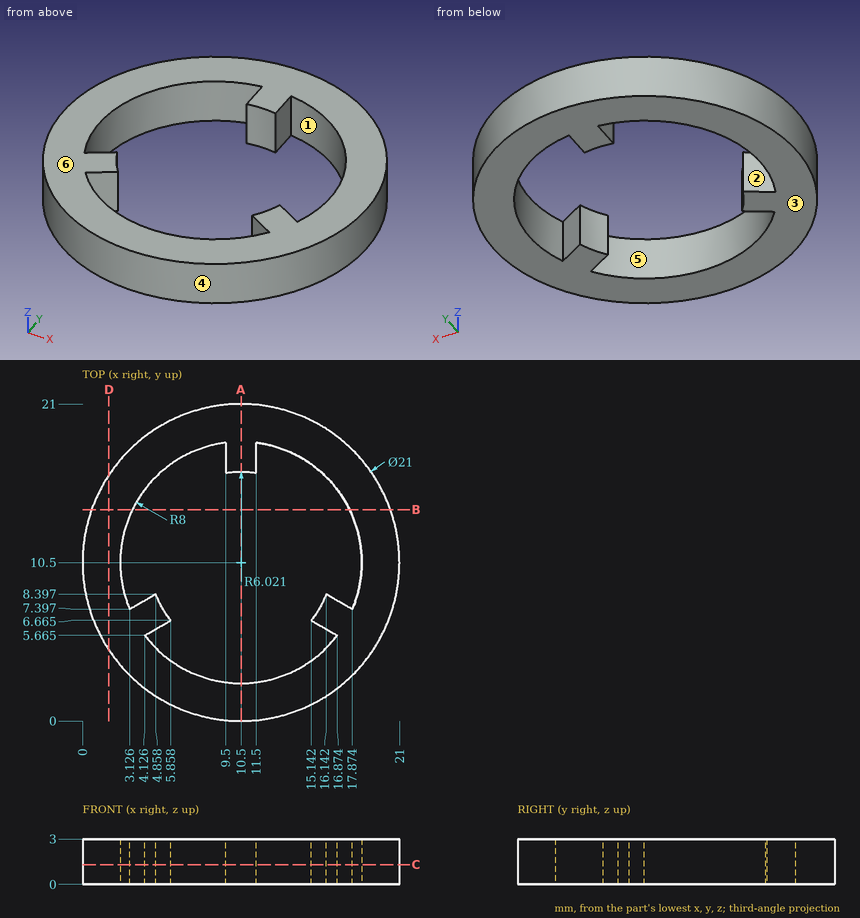
Job drawing, mm, ordinate dimensions from the low corner. One solid piece. A direction names the side the tool comes from. Round coordinates to 2 decimals unless told otherwise and drop trailing zeros. Loops run counter-clockwise (first coordinate to the right, second up) from the corner with the lowest first, then second, coordinate; pieces in that order, holes last.
(1) Cut at C-C (z = 1.3). Give the cut face in (x, y) (1 decimal).
(2) Wall check: line 1 along Y through (x, z) = (15.25, 1.85) (1 decimal); line 2 along X through (y, z) = (17.75, 0.6) (1 decimal); line 3 along Y through (x, z) = (4.75, 1.35) (1 decimal). Give the ranges that are in metal, low to high.
(3) Cut at B-B (y = 14). Give the cut face in (x, z).
(4) Cut at A-A (x = 10.5). Give the cut face in (y, z).
(5) Drop flat-ended pins along their axis: pin 1 (1.5 mm diameter, centred on x = 17, y = 14, fed in from +Z); pin 2 (1.6 mm diameter, centred on y = 18, z = 1, fed in from -X) (1 decimal); pin 3 (1 mm diameter, centred on y = 17.5, z = 1.5, fed in from +X) (1 decimal). Give the stop position or say it passes through.
(6) Two-plate mould, pull along X, no slides. Class the marked faces 1, 2, 3 and 4: +X half, -X half, draft (parallel to the pull), parting line (faces both ways), or undercut.
(7) Which spindle directions (+Z, -Z, +X, -X, +Y, -Y) get a long thin tool onto all of the face, cutting with end or side? Do the marked faces 5 and 6. Say none if no direction does.
(8) Cut at D-D (x = 1.75). Give the cut face in (y, z), plus the area to 3 significant figures.
Findings below:
1. outline: circle Ø21 at (10.5, 10.5); hole (3.1, 7.4) - (4.9, 8.4) arc R6 ccw to (5.9, 6.7) - (4.1, 5.7) arc R8 ccw to (16.9, 5.7) - (15.1, 6.7) arc R6 ccw to (16.1, 8.4) - (17.9, 7.4) arc R8 ccw to (11.5, 18.4) - (11.5, 16.4) arc R6 ccw to (9.5, 16.4) - (9.5, 18.4) arc R8 ccw to start
2. line 1: y = 1.1 to 4.1, 6.6 to 6.8, 16.9 to 19.9
2. line 2: x = 2.9 to 7.1, 9.5 to 11.5, 13.9 to 18.1
2. line 3: y = 1.7 to 4.9, 6 to 8.3, 16.1 to 19.3
3. outline: (0.6, 0) - (3.31, 0) - (3.31, 3) - (0.6, 3) - close; (17.69, 0) - (20.4, 0) - (20.4, 3) - (17.69, 3) - close
4. outline: (0, 0) - (2.5, 0) - (2.5, 3) - (0, 3) - close; (16.52, 0) - (21, 0) - (21, 3) - (16.52, 3) - close
5. pin 1: stops at z = 3
5. pin 2: stops at x = 2.4
5. pin 3: stops at x = 18.7
6. face 1: undercut
6. face 2: undercut
6. face 3: draft
6. face 4: parting line
7. face 5: +Z, -Z
7. face 6: +Z, +X, -X, +Y, -Y
8. outline: (4.7, 0) - (16.3, 0) - (16.3, 3) - (4.7, 3) - close
8. area: 34.8 mm2
